from build123d import *

# Parameters (mm, degrees)
ESQUISSE18_R        = 1.5
BOSS_EXTRU_18_DEPTH = 3


with BuildPart() as part:
    # Esquisse18 → Boss.-Extru.18 (new body)
    with BuildSketch(Plane.XY):
        with BuildLine():
            Line((83.995271076, 16.559954608), (97.025632531, 29.590316063))
            Line((97.025632531, 29.590316063), (97.025632531, 19.364814746))
            Line((97.025632531, 19.364814746), (91.995271076, 14.334453291))
            Line((91.995271076, 14.334453291), (91.995271076, 0.979857371))
            Line((91.995271076, 0.979857371), (92.123404239, 0.943388643))
            ThreePointArc((92.123404239, 0.943388643), (93.440738996, 1.864842376), (94.949542599, 2.419783395))
            ThreePointArc((94.949542599, 2.419783395), (95.094740148, 2.416733928), (95.221491727, 2.345842004))
            ThreePointArc((95.221491727, 2.345842004), (95.454932198, 2.119520802), (95.6812534, 1.886080331))
            ThreePointArc((95.6812534, 1.886080331), (95.752145324, 1.759328753), (95.755194791, 1.614131203))
            ThreePointArc((95.755194791, 1.614131203), (95.200253772, 0.1053276), (94.278800038, -1.212007157))
            ThreePointArc((94.278800038, -1.212007157), (94.201940613, -1.384508915), (94.243380312, -1.568755975))
            Line((94.243380312, -1.568755975), (94.308995173, -1.680100401))
            ThreePointArc((94.308995173, -1.680100401), (94.341055685, -1.73620681), (94.372614843, -1.792596749))
            ThreePointArc((94.372614843, -1.792596749), (94.511457628, -1.920608112), (94.699278246, -1.940296776))
            ThreePointArc((94.699278246, -1.940296776), (96.300850478, -1.800961813), (97.884983236, -2.074770594))
            ThreePointArc((97.884983236, -2.074770594), (98.009203269, -2.150010285), (98.083527395, -2.274780281))
            ThreePointArc((98.083527395, -2.274780281), (98.172532171, -2.587500427), (98.251811846, -2.902826406))
            ThreePointArc((98.251811846, -2.902826406), (98.249830264, -3.048042455), (98.179872405, -3.175311955))
            ThreePointArc((98.179872405, -3.175311955), (96.944877584, -4.204503695), (95.488207864, -4.884622193))
            ThreePointArc((95.488207864, -4.884622193), (95.33539477, -4.995583385), (95.279159072, -5.175865869))
            Line((95.279159072, -5.175865869), (95.280310995, -5.305100401))
            ThreePointArc((95.280310995, -5.305100401), (95.280023009, -5.369720233), (95.279159072, -5.434334932))
            ThreePointArc((95.279159072, -5.434334932), (95.33539477, -5.614617416), (95.488207864, -5.725578608))
            ThreePointArc((95.488207864, -5.725578608), (96.944877584, -6.405697106), (98.179872405, -7.434888846))
            ThreePointArc((98.179872405, -7.434888846), (98.249830264, -7.562158346), (98.251811846, -7.707374395))
            ThreePointArc((98.251811846, -7.707374395), (98.172532171, -8.022700374), (98.083527395, -8.33542052))
            ThreePointArc((98.083527395, -8.33542052), (98.009203269, -8.460190516), (97.884983236, -8.535430207))
            ThreePointArc((97.884983236, -8.535430207), (96.300850478, -8.809238989), (94.699278246, -8.669904025))
            ThreePointArc((94.699278246, -8.669904025), (94.511457628, -8.68959269), (94.372614843, -8.817604052))
            Line((94.372614843, -8.817604052), (94.308995173, -8.930100401))
            ThreePointArc((94.308995173, -8.930100401), (94.276435853, -8.985918824), (94.243380312, -9.041444826))
            ThreePointArc((94.243380312, -9.041444826), (94.201940613, -9.225691886), (94.278800038, -9.398193644))
            ThreePointArc((94.278800038, -9.398193644), (95.200253772, -10.715528401), (95.755194791, -12.224332004))
            ThreePointArc((95.755194791, -12.224332004), (95.752145324, -12.369529554), (95.6812534, -12.496281132))
            ThreePointArc((95.6812534, -12.496281132), (95.454932198, -12.729721603), (95.221491727, -12.956042805))
            ThreePointArc((95.221491727, -12.956042805), (95.094740148, -13.026934729), (94.949542599, -13.029984196))
            ThreePointArc((94.949542599, -13.029984196), (93.440738996, -12.475043177), (92.123404239, -11.553589444))
            ThreePointArc((92.123404239, -11.553589444), (91.950902481, -11.476730018), (91.76665542, -11.518169717))
            Line((91.76665542, -11.518169717), (91.655310995, -11.583784578))
            ThreePointArc((91.655310995, -11.583784578), (91.599204585, -11.61584509), (91.542814646, -11.647404249))
            ThreePointArc((91.542814646, -11.647404249), (91.414803284, -11.786247034), (91.39511462, -11.974067651))
            ThreePointArc((91.39511462, -11.974067651), (91.534449583, -13.575639883), (91.260640801, -15.159772642))
            ThreePointArc((91.260640801, -15.159772642), (91.185401111, -15.283992675), (91.060631115, -15.3583168))
            ThreePointArc((91.060631115, -15.3583168), (90.747910969, -15.447321577), (90.43258499, -15.526601252))
            ThreePointArc((90.43258499, -15.526601252), (90.287368941, -15.52461967), (90.160099441, -15.454661811))
            ThreePointArc((90.160099441, -15.454661811), (89.130907701, -14.219666989), (88.450789203, -12.762997269))
            ThreePointArc((88.450789203, -12.762997269), (88.339828011, -12.610184175), (88.159545526, -12.553948477))
            Line((88.159545526, -12.553948477), (88.030310995, -12.555100401))
            ThreePointArc((88.030310995, -12.555100401), (87.965691163, -12.554812414), (87.901076464, -12.553948477))
            ThreePointArc((87.901076464, -12.553948477), (87.72079398, -12.610184175), (87.609832788, -12.762997269))
            ThreePointArc((87.609832788, -12.762997269), (86.929714289, -14.219666989), (85.900522549, -15.454661811))
            ThreePointArc((85.900522549, -15.454661811), (85.77325305, -15.52461967), (85.628037, -15.526601252))
            ThreePointArc((85.628037, -15.526601252), (85.312711022, -15.447321577), (84.999990876, -15.3583168))
            ThreePointArc((84.999990876, -15.3583168), (84.875220879, -15.283992675), (84.799981189, -15.159772642))
            ThreePointArc((84.799981189, -15.159772642), (84.526172407, -13.575639883), (84.66550737, -11.974067651))
            ThreePointArc((84.66550737, -11.974067651), (84.645818706, -11.786247034), (84.517807344, -11.647404249))
            Line((84.517807344, -11.647404249), (84.405310995, -11.583784578))
            ThreePointArc((84.405310995, -11.583784578), (84.349492572, -11.551225258), (84.29396657, -11.518169717))
            ThreePointArc((84.29396657, -11.518169717), (84.10971951, -11.476730018), (83.937217751, -11.553589444))
            ThreePointArc((83.937217751, -11.553589444), (82.619882994, -12.475043177), (81.111079391, -13.029984196))
            ThreePointArc((81.111079391, -13.029984196), (80.965881842, -13.026934729), (80.839130263, -12.956042805))
            ThreePointArc((80.839130263, -12.956042805), (80.605689793, -12.729721603), (80.37936859, -12.496281132))
            ThreePointArc((80.37936859, -12.496281132), (80.308476666, -12.369529554), (80.3054272, -12.224332004))
            ThreePointArc((80.3054272, -12.224332004), (80.860368218, -10.715528401), (81.781821952, -9.398193644))
            ThreePointArc((81.781821952, -9.398193644), (81.858681377, -9.225691886), (81.817241678, -9.041444826))
            Line((81.817241678, -9.041444826), (81.751626818, -8.930100401))
            ThreePointArc((81.751626818, -8.930100401), (81.719566305, -8.873993991), (81.688007147, -8.817604052))
            ThreePointArc((81.688007147, -8.817604052), (81.549164362, -8.68959269), (81.361343744, -8.669904025))
            ThreePointArc((81.361343744, -8.669904025), (79.759771513, -8.809238989), (78.175638754, -8.535430207))
            ThreePointArc((78.175638754, -8.535430207), (78.051418721, -8.460190516), (77.977094596, -8.33542052))
            ThreePointArc((77.977094596, -8.33542052), (77.888089819, -8.022700374), (77.808810144, -7.707374395))
            ThreePointArc((77.808810144, -7.707374395), (77.810791726, -7.562158346), (77.880749585, -7.434888846))
            ThreePointArc((77.880749585, -7.434888846), (79.115744406, -6.405697106), (80.572414127, -5.725578608))
            ThreePointArc((80.572414127, -5.725578608), (80.725227221, -5.614617416), (80.781462919, -5.434334932))
            Line((80.781462919, -5.434334932), (80.780310995, -5.305100401))
            ThreePointArc((80.780310995, -5.305100401), (80.780598982, -5.240480568), (80.781462919, -5.175865869))
            ThreePointArc((80.781462919, -5.175865869), (80.725227221, -4.995583385), (80.572414127, -4.884622193))
            ThreePointArc((80.572414127, -4.884622193), (79.115744406, -4.204503695), (77.880749585, -3.175311955))
            ThreePointArc((77.880749585, -3.175311955), (77.810791726, -3.048042455), (77.808810144, -2.902826406))
            ThreePointArc((77.808810144, -2.902826406), (77.888089819, -2.587500427), (77.977094596, -2.274780281))
            ThreePointArc((77.977094596, -2.274780281), (78.051418721, -2.150010285), (78.175638754, -2.074770594))
            ThreePointArc((78.175638754, -2.074770594), (79.759771513, -1.800961813), (81.361343744, -1.940296776))
            ThreePointArc((81.361343744, -1.940296776), (81.549164362, -1.920608112), (81.688007147, -1.792596749))
            Line((81.688007147, -1.792596749), (81.751626818, -1.680100401))
            ThreePointArc((81.751626818, -1.680100401), (81.784186138, -1.624281977), (81.817241678, -1.568755975))
            ThreePointArc((81.817241678, -1.568755975), (81.858681377, -1.384508915), (81.781821952, -1.212007157))
            ThreePointArc((81.781821952, -1.212007157), (80.860368218, 0.1053276), (80.3054272, 1.614131203))
            ThreePointArc((80.3054272, 1.614131203), (80.308476666, 1.759328753), (80.37936859, 1.886080331))
            ThreePointArc((80.37936859, 1.886080331), (80.605689793, 2.119520802), (80.839130263, 2.345842004))
            ThreePointArc((80.839130263, 2.345842004), (80.965881842, 2.416733928), (81.111079391, 2.419783395))
            ThreePointArc((81.111079391, 2.419783395), (82.619882994, 1.864842376), (83.937217751, 0.943388643))
            Line((83.937217751, 0.943388643), (83.995271076, 0.970909453))
            Line((83.995271076, 0.970909453), (83.995271076, 16.559954608))
        make_face()
        with Locations((88.030310995, -5.305100401)):
            Circle(ESQUISSE18_R, mode=Mode.SUBTRACT)
        with Locations((88.030310995, 4.590763304)):
            Circle(ESQUISSE18_R, mode=Mode.SUBTRACT)
    extrude(amount=BOSS_EXTRU_18_DEPTH)


solid = part.part
The listing builds one solid part. Answer for the finished solid, in the listing's coordinates (mm). A direction names the side the tool comes from. Coordinates: 2 decimals unless noted, no trailing zeros. Write each loop counter-clockwise with the first axis right and the second up, starting at its lowest first coordinate (ties: lowest second). Pieces come first, ordered by that corner, then holes. Notation, with made-up numbers: (11.25, -27.5) - (18.25, -27.5) arc R16 cw to (18.25, -4.5) - close; hole circle Ø10 at (88, 80.25). An arc over 180 degrees is marked (long way). Return JSON: item names as keys, results as strings.
1. Consider line 1 along Y through (x, z) = (87, 0.8); line 2 along Y through (x, z) = (94.5, 0.7); line 3 along Y through (x, z) = (88.25, 0.65). Determine where each line is inside the solid, lowest interval first.
Final values:
{"line 1": "-14.11 to -6.4, -4.21 to 3.5, 5.68 to 19.56", "line 2": "-12.91 to -9.65, -8.7 to -1.92, -0.96 to 2.3, 16.84 to 27.06", "line 3": "-12.57 to -6.79, -3.82 to 3.11, 6.07 to 20.81"}
2. This flat-tipped pin is pushed along its axis until it touches: pin 1 Ø1.5 at (y, z) = (25, 1) entering from +X. Where does it stop, or does it pass through?
Final values:
{"pin 1": "x = 97.03"}
3. The part is cut by section A-A on x = 96.5. Determine the outline of the cut face in (y, z), then the cut area to 3 significant figures.
Final values:
{"outline": "(-8.8, 0) - (-6.15, 0) - (-6.15, 3) - (-8.8, 3) - close; (-4.46, 0) - (-1.81, 0) - (-1.81, 3) - (-4.46, 3) - close; (18.84, 0) - (29.06, 0) - (29.06, 3) - (18.84, 3) - close", "area": "46.6 mm^2"}
4. For a pull along Y with two mould halves and no side action, classify faces 5 (the face through (79.097, -6.418, 1.479)), 6 (the face through (88, 2, 0)), 7 (the face through (86.94, -14.2, 1.48)) as +Y half, -Y half, draft (parallel to the pull), parting line (faces both ways), or undercut.
Final values:
{"face 5": "undercut", "face 6": "draft", "face 7": "-Y half"}
5. The part is cut by section D-D on z = 1.8. Count the separate pieces of the cut face and the enclosed holes in it, then the cut area to 3 significant figures.
Final values:
{"separate pieces": "1", "enclosed holes": "2", "area": "432 mm^2"}
6. The part is cut by section B-B on x = 79. Determine the outline of the cut face in (y, z), then the cut area to 3 significant figures.
Final values:
{"outline": "(-8.73, 0) - (-6.48, 0) - (-6.48, 3) - (-8.73, 3) - close; (-4.13, 0) - (-1.88, 0) - (-1.88, 3) - (-4.13, 3) - close", "area": "13.5 mm^2"}
7. The part is cut by section C-C on y = 10.5. Determine the outline of the cut face in (x, z).
Final values:
{"outline": "(84, 0) - (92, 0) - (92, 3) - (84, 3) - close"}
8. Which of the six approach directions +Z, -Z, +X, -X, +Y, -Y give full straight-line access (tool end or side, diameter ignored) to faces 1 (the face through (96.926, -6.394, 1.479)), 2 (the face through (93.421, 1.854, 1.479)), 3 (the face through (82.64, -12.465, 1.479)), 4 (the face through (97.026, 25, 1))?
Final values:
{"face 1": "+Z, -Z, +X", "face 2": "+Z, -Z", "face 3": "+Z, -Z, -Y", "face 4": "+Z, -Z, +X, +Y"}
